```python
from build123d import *

# Parameters (mm, degrees)
CYLINDER_R     = 4
CYLINDER_DEPTH = 40
TUBE_R         = 26
TUBE_R_2       = 23.5
TUBE_DEPTH     = 40
CHAMFER_SIZE   = 1


with BuildPart() as cylinder:
    # Cylinder → Cylinder (new body)
    with BuildSketch(Plane.XY.offset(40)):
        Circle(CYLINDER_R)
    extrude(amount=CYLINDER_DEPTH)


with BuildPart() as tube:
    # Tube → Tube (new body)
    with BuildSketch(Plane.XY):
        Circle(TUBE_R)
        Circle(TUBE_R_2, mode=Mode.SUBTRACT)
    extrude(amount=TUBE_DEPTH)


with BuildPart() as chamfer_body:
    # Cone → Cone (revolve)
    with BuildSketch(Plane(origin=(0, 0, 40), x_dir=(1, 0, 0), z_dir=(0, -1, 0))):
        Polygon((0, 0), (26, 0), (6, 40), (0, 40), align=None)
    revolve(axis=Axis((0, 0, 40), (0, 0, 1)))

    # Fusion: union Tube
    add(tube.part)

    # Cut: cut Cylinder
    add(cylinder.part, mode=Mode.SUBTRACT)

    # Chamfer
    chamfer_edges = [chamfer_body.edges().sort_by_distance(p)[0] for p in [
        (-26, 0, 0),
        (-23.5, 0, 0),
    ]]
    chamfer(chamfer_edges, length=CHAMFER_SIZE)


solid = chamfer_body.part
```
Check sheet for the modelled part. Datum: model origin and axes. Units: mm. A direction names the side the tool comes from. Give positions to 0.01 mm unless a question says otherwise; leave off trailing zeros. Order: outer loops, then holes, each group sorted by start corner. A loop starts at its lowest first (then second) coordinate and runs counter-clockwise, first axis right, second up. Notation, with made-up numbers: (89.25, 51.25) -> (137.25, 51.25) arc R15 ccw to (137.25, 57.25) -> close; hole circle Ø5 at (65, 25). An arc over 180 degrees is marked (long way). Return JSON: item names as keys, results as strings.
1. Set-up check for faces 1 (the flat face through (0, -5, 40)), 2 (the flat face through (18, -17, 0)): record each of +Z, -Z, +X, -X, +Y, -Y from which the full face is reachable in a straight line by a thin tool's end or side.
From the geometry:
{"face 1": "-Z", "face 2": "-Z, +X, -X, +Y, -Y"}
2. Go/stop test with flat-tipped pins: P1, Ø1, axis at y = -6, z = 36.5, coming from the +X side; P2, Ø2, axis at x = 0, z = 52, coming from the +Y side; P3, Ø12, axis at y = 17.5, z = 61.5, coming from the +X side. Record where each tip stops, or that it passes through.
From the geometry:
{"P1": "x = 25.41", "P2": "y = 20.5", "P3": "x = 11.39"}
3. Material ranges on probe 1 along Y at (x, z) = (0.5, 31.5); probe 2 along X at (y, z) = (-16, 5.5), recorded low to high. Write a range as [from, to].
From the geometry:
{"probe 1": "[-26, -23.49], [23.49, 26]", "probe 2": "[-20.49, -17.21], [17.21, 20.49]"}
4. Cross-section at D-D, the plane z = 31. Record the cut outline in (x, y), plus the area to 3 significant figures.
From the geometry:
{"outline": "circle Ø52 at (0, 0); hole circle Ø47 at (0, 0)", "area": "389 mm^2"}
5. Mould release check, pull along Y, two halves, no side actions. Record for faces 3 (the flat face through (-1.42, -3.92, 80)), 4 (the cylindrical face through (-20.633, -15.821, 20.227)), 5 (the cylindrical face through (22.4, 7.1, 20.2)): +Y half, -Y half, draft (parallel to the pull), parting line (faces both ways), or undercut.
From the geometry:
{"face 3": "draft", "face 4": "parting line", "face 5": "undercut"}
6. Cross-section at A-A, the plane y = 0. Record the cut outline in (x, z), plus the area to 3 significant figures.
From the geometry:
{"outline": "(-26, 1) -> (-25, 0) -> (-24.5, 0) -> (-23.5, 1) -> (-23.5, 40) -> (-4, 40) -> (-4, 80) -> (-6, 80) -> (-26, 40) -> close; (4, 40) -> (23.5, 40) -> (23.5, 1) -> (24.5, 0) -> (25, 0) -> (26, 1) -> (26, 40) -> (6, 80) -> (4, 80) -> close", "area": "1,160 mm^2"}
7. Cross-section at C-C, the plane z = 62. Record the cut outline in (x, y).
From the geometry:
{"outline": "circle Ø30 at (0, 0); hole circle Ø8 at (0, 0)"}
